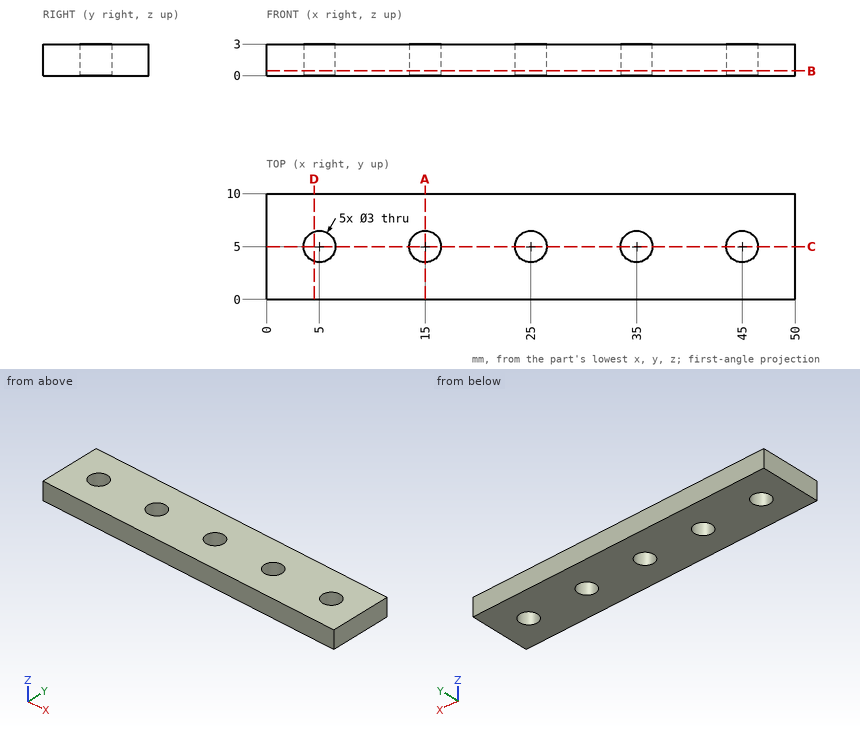
Design review of the part shown in the three views and the two pictorial views. Dimensions are in mm from the part's minimum x, y and z. Round coordinates to 2 decimals unless told otherwise and drop trailing zeros. Write each loop counter-clockwise with the first axis right and the second up, starting at its lowest first coordinate (ties: lowest second). Pieces come first, ordered by that corner, then holes. Notation, with made-up numbers: (-29, 80.5) -> (-14, 80.5) arc R17 cw to (-14, 94.5) -> close; hole circle Ø9 at (-10, 22). An arc over 180 degrees is marked (long way). Write item = value, one per line. Start each with the question number.
1) Clearance check with a flat-ended pin moving along its axis: pin 1 (5 mm diameter, centred on x = 15, y = 5, fed in from +Z). State where the tip first meets the part, or that it passes through.
2) Wall thickness on probe 1 along X at (y, z) = (5, 1); probe 2 along Y at (x, z) = (35, 2.2); probe 3 along X at (y, z) = (4.25, 2.35): over which ranges is each line inside the solid? List them lowest first. Write a range as from..to.
3) Take a section at C-C, the plane y = 5. State the section outline as (x, z) points.
4) Take a section at B-B, the plane z = 0.45. State the section outline as (x, y) points.
5) Take a section at A-A, the plane x = 15. State the section outline as (y, z) points, plus the area to 3 significant figures.
6) Take a section at D-D, the plane x = 4.5. State the section outline as (y, z) points.
Results list:
q1.pin_1 = 3
q2.probe_1 = 0..3.5, 6.5..13.5, 16.5..23.5, 26.5..33.5, 36.5..43.5, 46.5..50
q2.probe_2 = 0..3.5, 6.5..10
q2.probe_3 = 0..3.7, 6.3..13.7, 16.3..23.7, 26.3..33.7, 36.3..43.7, 46.3..50
q3.outline = (0, 0) -> (3.5, 0) -> (3.5, 3) -> (0, 3) -> close; (6.5, 0) -> (13.5, 0) -> (13.5, 3) -> (6.5, 3) -> close; (16.5, 0) -> (23.5, 0) -> (23.5, 3) -> (16.5, 3) -> close; (26.5, 0) -> (33.5, 0) -> (33.5, 3) -> (26.5, 3) -> close; (36.5, 0) -> (43.5, 0) -> (43.5, 3) -> (36.5, 3) -> close; (46.5, 0) -> (50, 0) -> (50, 3) -> (46.5, 3) -> close
q4.outline = (0, 0) -> (50, 0) -> (50, 10) -> (0, 10) -> close; hole circle Ø3 at (5, 5); hole circle Ø3 at (15, 5); hole circle Ø3 at (25, 5); hole circle Ø3 at (35, 5); hole circle Ø3 at (45, 5)
q5.outline = (0, 0) -> (3.5, 0) -> (3.5, 3) -> (0, 3) -> close; (6.5, 0) -> (10, 0) -> (10, 3) -> (6.5, 3) -> close
q5.area = 21.0 mm²
q6.outline = (0, 0) -> (3.59, 0) -> (3.59, 3) -> (0, 3) -> close; (6.41, 0) -> (10, 0) -> (10, 3) -> (6.41, 3) -> close
